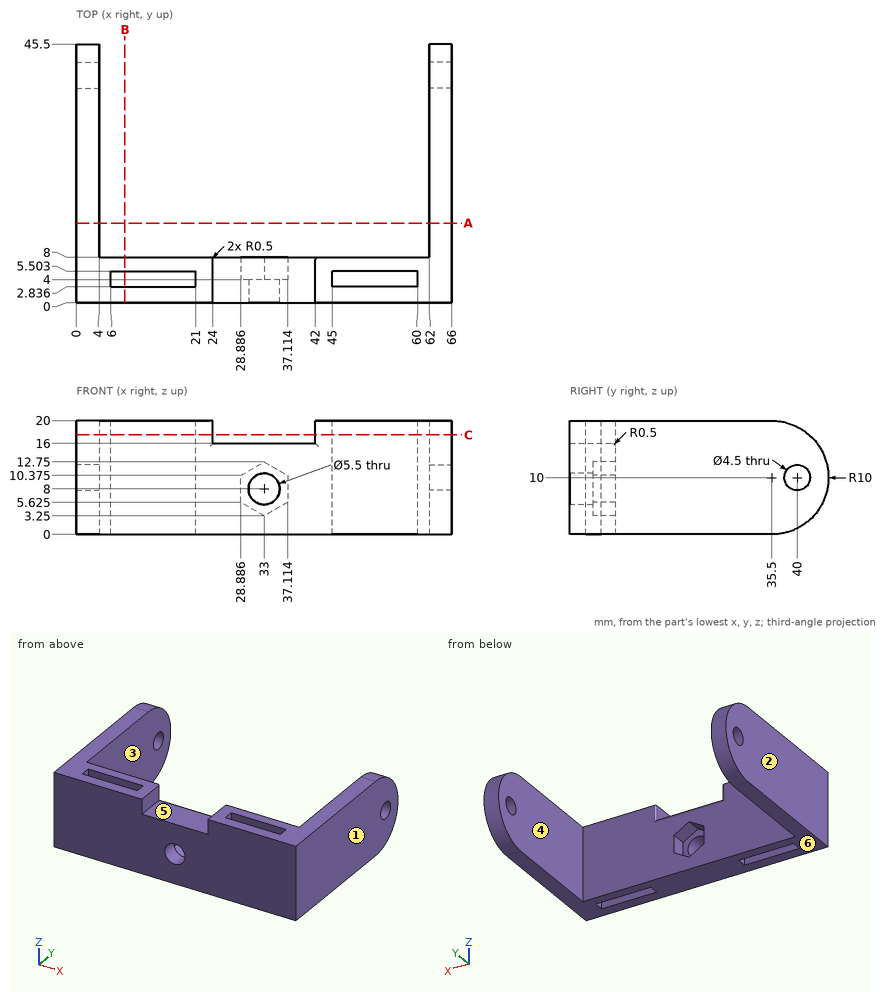
Check sheet for the drawn part. Datum: minimum x, y, z corner. Units: mm. A direction names the side the tool comes from. Round coordinates to 2 decimals unless told otherwise and drop trailing zeros. Order: outer loops, then holes, each group sorted by start corner. A loop starts at its lowest first (then second) coordinate and runs counter-clockwise, first axis right, second up. Notation, with made-up numbers: (-6, 81) -> (40, 81) arc R20 ccw to (40, 88) -> close; hole circle Ø7 at (-19.75, 25.25). An arc over 180 degrees is marked (long way). Use CSV: the item, a comma, the result in double quotes.
(1) Cross-section at B-B (x = 8.5). Record the boundary of the cut face in (y, z).
Worked out:
outline,"(0, 0) -> (2.84, 0) -> (2.84, 20) -> (0, 20) -> close; (5.5, 0) -> (8, 0) -> (8, 20) -> (5.5, 20) -> close"
(2) Cross-section at C-C (z = 17.5). Record the boundary of the cut face in (x, y) (1 decimal), and give its area (3 significant figures).
Worked out:
outline,"(0, 0) -> (24, 0) -> (24, 7.5) arc R0.5 ccw to (23.5, 8) -> (4, 8) -> (4, 42.1) -> (0, 42.1) -> close; (42, 0) -> (66, 0) -> (66, 42.1) -> (62, 42.1) -> (62, 8) -> (42.5, 8) arc R0.5 ccw to (42, 7.5) -> close; hole (6, 2.8) -> (21, 2.8) -> (21, 5.5) -> (6, 5.5) -> close; hole (45, 2.8) -> (60, 2.8) -> (60, 5.5) -> (45, 5.5) -> close"
area,"577 mm²"
(3) Cross-section at A-A (y = 14). Record the boundary of the cut face in (x, z), and give its area (3 significant figures).
Worked out:
outline,"(0, 0) -> (4, 0) -> (4, 20) -> (0, 20) -> close; (62, 0) -> (66, 0) -> (66, 20) -> (62, 20) -> close"
area,"160 mm²"
(4) Material ranges on line 1 along X through (y, z) = (3.5, 3.5); line 2 along Y through (x, z) = (52, 11.25); line 3 along X through (y, z) = (14, 2.75), recorded low to high. Write a range as from..to.
Worked out:
line 1,"0..6, 21..45, 60..66"
line 2,"0..2.84, 5.5..8"
line 3,"0..4, 62..66"
(5) Draft check along X on the marked faces 1, 2 and 3. Enter one of: pulls with the +X half, pulls with the -X half, needs draft (parallel to the pull), parting line crosses it, or undercut.
Worked out:
face 1,"pulls with the +X half"
face 2,"pulls with the -X half"
face 3,"undercut"
(6) Depth check by flat-ended pin: pin 1 (2 mm diameter, centred on x = 34, y = 3.5, fed in from +Z); pin 2 (9 mm diameter, centred on x = 33, z = 8.5, fed in from +Y); pin 3 (4 mm diameter, centred on y = 40, z = 10, fed in from +X). Enter the tip coordinate at first touch or a pass-through.
Worked out:
pin 1,"z = 16"
pin 2,"y = 8"
pin 3,"through"
(7) Tool access check on the marked faces 4, 5 and 6. Record the directions out of +Z, -Z, +X, -X, +Y, -Y that give a thin tool (end or side, any length) a straight path to the whole face; none if there is none.
Worked out:
face 4,"+Z, -Z, +Y"
face 5,"+Z, +Y, -Y"
face 6,"-Z, +X, -X, +Y, -Y"
